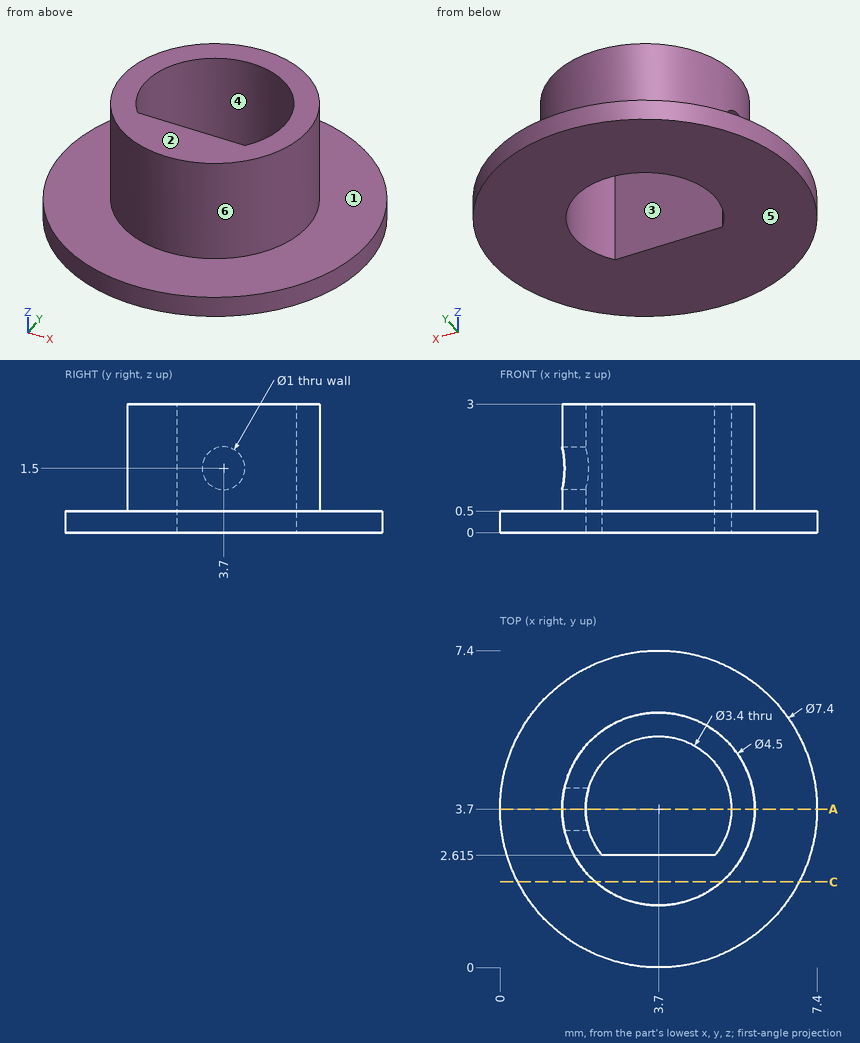
Geometry check sheet. Reference: drawing and pictorial views, mm from the part's lowest x, y, z. A direction names the side the tool comes from. Give positions to 0.01 mm unless a question says otherwise; leave off trailing zeros. Order: outer loops, then holes, each group sorted by start corner. A loop starts at its lowest first (then second) coordinate and runs counter-clockwise, first axis right, second up. Notation, with made-up numbers: M 42,73.5 L 67,73.5 A16 ccw 67,90.5 Z; hole C 79.25,33.25 d8. An arc over 180 degrees is marked long. Answer in a Markdown table with one row per item.
1) Release check for a two-part mould opening along Y. For the marked faces 4, 5 and 6 record: +Y half, -Y half, draft (parallel to the pull), parting line (faces both ways), or undercut.
Filled sheet:
| item | result |
|---|---|
| face 4 | undercut |
| face 5 | draft |
| face 6 | parting line |
2) Cross-section at A-A, the plane y = 3.7. Enter the section's corners in (x, z).
Filled sheet:
| item | result |
|---|---|
| outline | M 0,0 L 2,0 L 2,1 L 1.45,1 L 1.45,0.5 L 0,0.5 Z; M 1.45,2 L 2,2 L 2,3 L 1.45,3 Z; M 5.4,0 L 7.4,0 L 7.4,0.5 L 5.95,0.5 L 5.95,3 L 5.4,3 Z |
3) Gauge pin test, flat ends, axial feed: P1, Ø1.5, axis at x = 2.5, z = 1.5, coming from the -Y side (1 decimal); P2, Ø4, axis at x = 3.7, y = 3.7, coming from the -Z side; P3, Ø1.3, axis at x = 3, z = 1.5, coming from the +Y side; P4, Ø1, axis at y = 6, z = 1.5, coming from the -X side. Record the tip position at first contact, or that the pin passes through.
Filled sheet:
| item | result |
|---|---|
| P1 | stops at y = 1.5 |
| P2 | stops at z = 0 |
| P3 | stops at y = 5.95 |
| P4 | stops at x = 2.35 |
4) Access from +Z, -Z, +X, -X, +Y, -Y to the whole of each face (thin tool, end or side, straight path). Record for the marked faces 1, 2 and 3.
Filled sheet:
| item | result |
|---|---|
| face 1 | +Z |
| face 2 | +Z, +X, -X, +Y, -Y |
| face 3 | +Z, -Z |
5) Cross-section at C-C, the plane y = 2. Enter the section's corners in (x, z).
Filled sheet:
| item | result |
|---|---|
| outline | M 0.41,0 L 6.99,0 L 6.99,0.5 L 5.17,0.5 L 5.17,3 L 2.23,3 L 2.23,0.5 L 0.41,0.5 Z |
6) Thickness scan on L1, parallel to X at y = 3.7, z = 0.8; L2, parallel to Z at x = 1.6, y = 3.7; L3, parallel to Z at x = 2.5, y = 1.75. Record the ranges inside material, lowest first. Write a range as [from, to].
Filled sheet:
| item | result |
|---|---|
| L1 | x = [1.45, 2], [5.4, 5.95] |
| L2 | z = [0, 1], [2, 3] |
| L3 | z = [0, 0.5] |
